Read the model definition and answer for the solid it produces. Units are mm, in the model's axes. A direction names the side the tool comes from. Round coordinates to 2 decimals unless told otherwise and drop trailing zeros. Order: outer loops, then holes, each group sorted by start corner. A loop starts at its lowest first (then second) coordinate and runs counter-clockwise, first axis right, second up. Notation, with made-up numbers: (68, 37.25) -> (89, 37.25) arc R11 cw to (89, 54.25) -> close; hole circle Ø7 at (63, -32.75). An arc over 180 degrees is marked (long way). Answer as a JSON object with one key per item and string values. Group by question number.
Item 1: Given P1, Ø11.5, axis at x = 18, z = -9, coming from the +Y side; P2, Ø6, axis at x = 160.5, z = -59.5, coming from the -Y side, each flat-ended and moving along its own axis, determine where each tip first touches the part or whether it passes through.
Item 2: For faces 1 (the flat face through (16.328, 2.421, -36.696)), 2 (the cylindrical face through (139.773, 10.988, -4.93)), 3 (the flat face through (178, 13, -9)), determine the directions among +Z, -Z, +X, -X, +Y, -Y from which every point of the face is accessible in a straight line to the end or side of a thin tool.
Item 3: The mould has two halves that part along X. Classify faces 4 (the flat face through (3, 15.2, -103.9)), 5 (the flat face through (16, 12.4, -34)), 6 (the flat face through (97, 0, -30)): pulls with the +X half, pulls with the -X half, needs draft (parallel to the pull), parting line crosses it, or undercut.
Item 4: Section C-C, the plane x = 68 is taken. Write down the section's boundary in (y, z).
Item 5: Section B-B, the plane y = 17.5 is taken. Count the separate pieces of the cut face and the enclosed holes in it, plus the area to 3 significant figures.
Item 6: Section D-D, the plane z = -73 is taken. Write down the section's boundary in (x, y) (3 decimals), plus the area to 3 significant figures.
Item 7: Section A-A, the plane x = 178 is taken. Write down the section's boundary in (y, z), plus the area to 3 significant figures.
Item 8: Consider probe 1 along X at (y, z) = (15, -53); probe 2 along X at (y, z) = (20, -98); probe 3 along Z at (x, y) = (138.5, 2.25). Determine where each line is inside the solid, lowest interval first. Write a range as from..to.
from build123d import *

# Parameters (mm, degrees)
SKETCH1_W            = 197
SKETCH1_H            = 107
BOSS_EXTRUDE1_DEPTH  = 30
SKETCH4_W            = 182
SKETCH4_H            = 45
CUT_EXTRUDE2_DEPTH   = 10
BOSS_EXTRUDE11_DEPTH = 10
CUT_EXTRUDE28_DEPTH  = 14.5
SKETCH9_R            = 8
CUT_EXTRUDE6_DEPTH   = 171
SKETCH10_R           = 9.5
CUT_EXTRUDE7_DEPTH   = 1.5
SKETCH11_R           = 4.95
CUT_EXTRUDE8_DEPTH   = 17.6
SKETCH41_R           = 2.9
CUT_EXTRUDE21_DEPTH  = 7
CUT_EXTRUDE22_DEPTH  = 10
CUT_EXTRUDE23_DEPTH  = 10
CUT_EXTRUDE29_DEPTH  = 14.5
CUT_EXTRUDE36_DEPTH  = 55.4
SKETCH90_R           = 6.35
CUT_EXTRUDE38_DEPTH  = 17
SKETCH91_W           = 141.2
SKETCH91_H           = 21.2
CUT_EXTRUDE39_DEPTH  = 2.3
CUT_EXTRUDE40_DEPTH  = 227.181343174


with BuildPart() as part:
    # Sketch1 → Boss-Extrude1 (new body)
    with BuildSketch(Plane(origin=(0, 0, 0), x_dir=(1, 0, 0), z_dir=(0, 1, 0))):
        with Locations((98.5, 53.5)):
            Rectangle(SKETCH1_W, SKETCH1_H)
    extrude(amount=BOSS_EXTRUDE1_DEPTH)

    # Sketch4 → Cut-Extrude2 (cut)
    with BuildSketch(Plane(origin=(0, 0, 0), x_dir=(1, 0, 0), z_dir=(0, 1, 0))):
        with Locations((98.5, 53.5)):
            Rectangle(SKETCH4_W, SKETCH4_H)
    extrude(amount=CUT_EXTRUDE2_DEPTH, mode=Mode.SUBTRACT)

    # Sketch53 → Boss-Extrude11 (add)
    with BuildSketch(Plane(origin=(0, 10, 0), x_dir=(-1, 0, 0), z_dir=(0, -1, 0))):
        Polygon((-7.5, 51), (-7.5, 31), (-38.5, 31), align=None)
        Polygon((-7.5, 56), (-7.5, 76), (-38.5, 76), align=None)
    extrude(amount=BOSS_EXTRUDE11_DEPTH)

    # Izq → Cut-Extrude28 (cut)
    with BuildSketch(Plane(origin=(0, 27.358390683, -11.62731604), x_dir=(1, 0, 0), z_dir=(0, 0.9203309184584746, -0.3911406403448515))):
        Polygon((7.5, 48.213835991), (38.5, 69.945149803), (7.5, 69.945149803), align=None)
    extrude(amount=-CUT_EXTRUDE28_DEPTH, mode=Mode.SUBTRACT)

    # Sketch9 → Cut-Extrude6 (cut)
    with BuildSketch(Plane(origin=(0, 30, 0), x_dir=(1, 0, 0), z_dir=(0, 1, 0))):
        with Locations(Location((15.45, 53.5, 0), (0, 0, 270))):
            Circle(SKETCH9_R)
    extrude(amount=-CUT_EXTRUDE6_DEPTH, mode=Mode.SUBTRACT)

    # Sketch10 → Cut-Extrude7 (cut)
    with BuildSketch(Plane(origin=(0, 30, 0), x_dir=(1, 0, 0), z_dir=(0, 1, 0))):
        with Locations(Location((15.45, 53.5, 0), (0, 0, 270))):
            Circle(SKETCH10_R)
    extrude(amount=-CUT_EXTRUDE7_DEPTH, mode=Mode.SUBTRACT)

    # Sketch11 → Cut-Extrude8 (cut)
    with BuildSketch(Plane(origin=(0, 30, 0), x_dir=(1, 0, 0), z_dir=(0, 1, 0))):
        with Locations(Location((15.45, 72.905102572, 0), (0, 0, 270))):
            Circle(SKETCH11_R)
        with Locations(Location((15.45, 34.094897428, 0), (0, 0, 270))):
            Circle(SKETCH11_R)
    extrude(amount=-CUT_EXTRUDE8_DEPTH, mode=Mode.SUBTRACT)

    # Sketch41 → Cut-Extrude21 (cut)
    with BuildSketch(Plane(origin=(0, 0, 0), x_dir=(1, 0, 0), z_dir=(0, 1, 0))):
        with Locations(Location((138.5, 9, 0), (0, 0, 90))):
            Circle(SKETCH41_R)
        with Locations(Location((138.5, 98, 0), (0, 0, 90))):
            Circle(SKETCH41_R)
    extrude(amount=CUT_EXTRUDE21_DEPTH, mode=Mode.SUBTRACT)

    # Sketch42 → Cut-Extrude22 (cut)
    with BuildSketch(Plane.XY):
        with BuildLine():
            Line((141.261527075, 12.77273886), (151, 12.77273886))
            ThreePointArc((151, 12.77273886), (152.77273886, 11), (151, 9.22726114))
            Line((151, 9.22726114), (141.261527075, 9.27273886))
            ThreePointArc((141.261527075, 9.27273886), (139.77273886, 11.02273886), (141.261527075, 12.77273886))
        make_face()
    extrude(amount=-CUT_EXTRUDE22_DEPTH, mode=Mode.SUBTRACT)

    # Sketch43 → Cut-Extrude23 (cut)
    with BuildSketch(Plane(origin=(0, 0, -107), x_dir=(-1, 0, 0), z_dir=(0, 0, -1))):
        with BuildLine():
            Line((-55.7, 12.8), (-46, 12.8))
            ThreePointArc((-46, 12.8), (-44.2, 11), (-46, 9.2))
            Line((-46, 9.2), (-55.7, 9.2))
            ThreePointArc((-55.7, 9.2), (-57.5, 11), (-55.7, 12.8))
        make_face()
    extrude(amount=-CUT_EXTRUDE23_DEPTH, mode=Mode.SUBTRACT)

    # Der → Cut-Extrude29 (cut)
    with BuildSketch(Plane(origin=(0, -11.159343568, -4.742721016), x_dir=(1, 0, 0), z_dir=(0, 0.9203309184584747, 0.3911406403448517))):
        Polygon((7.5, 50.261572284), (38.5, 28.530258472), (7.5, 28.530258472), align=None)
    extrude(amount=-CUT_EXTRUDE29_DEPTH, mode=Mode.SUBTRACT)

    # Sketch85 → Cut-Extrude36 (cut)
    with BuildSketch(Plane(origin=(0, 30, 0), x_dir=(1, 0, 0), z_dir=(0, 1, 0))):
        Polygon((0, 100.9), (6.1, 107), (0, 107), align=None)
        Polygon((0, 0), (6.1, 0), (0, 6.1), align=None)
        Polygon((197, 6.1), (190.9, 0), (197, 0), align=None)
        Polygon((197, 107), (190.9, 107), (197, 100.9), align=None)
    extrude(amount=-CUT_EXTRUDE36_DEPTH, mode=Mode.SUBTRACT)

    # Sketch90 → Cut-Extrude38 (cut)
    with BuildSketch(Plane(origin=(0, 30, 0), x_dir=(1, 0, 0), z_dir=(0, 1, 0))):
        with Locations(Location((18, 9, 0), (0, 0, 270))):
            Circle(SKETCH90_R)
        with Locations(Location((98, 9, 0), (0, 0, 270))):
            Circle(SKETCH90_R)
        with Locations(Location((178, 9, 0), (0, 0, 270))):
            Circle(SKETCH90_R)
        with Locations(Location((98, 98, 0), (0, 0, 270))):
            Circle(SKETCH90_R)
        with Locations(Location((178, 98, 0), (0, 0, 270))):
            Circle(SKETCH90_R)
        with Locations(Location((18, 98, 0), (0, 0, 270))):
            Circle(SKETCH90_R)
    extrude(amount=-CUT_EXTRUDE38_DEPTH, mode=Mode.SUBTRACT)

    # Sketch91 → Cut-Extrude39 (cut)
    with BuildSketch(Plane(origin=(0, 30, 0), x_dir=(1, 0, 0), z_dir=(0, 1, 0))):
        with BuildLine():
            Line((42.6, 66.5), (182.6, 66.5))
            ThreePointArc((182.6, 66.5), (184.721320344, 65.621320344), (185.6, 63.5))
            Line((185.6, 63.5), (185.6, 43.5))
            ThreePointArc((185.6, 43.5), (184.721320344, 41.378679656), (182.6, 40.5))
            Line((182.6, 40.5), (42.6, 40.5))
            ThreePointArc((42.6, 40.5), (40.478679656, 41.378679656), (39.6, 43.5))
            Line((39.6, 43.5), (39.6, 63.5))
            ThreePointArc((39.6, 63.5), (40.478679656, 65.621320344), (42.6, 66.5))
        make_face()
        with Locations((112.6, 53.5)):
            Rectangle(SKETCH91_W, SKETCH91_H, mode=Mode.SUBTRACT)
    extrude(amount=-CUT_EXTRUDE39_DEPTH, mode=Mode.SUBTRACT)

    # Sketch93 → Cut-Extrude40 (cut, through all)
    with BuildSketch(Plane(origin=(0, 30, 0), x_dir=(1, 0, 0), z_dir=(0, 1, 0))):
        with BuildLine():
            Line((45.1, 43.5), (180.1, 43.5))
            ThreePointArc((180.1, 43.5), (181.867766953, 44.232233047), (182.6, 46))
            Line((182.6, 46), (182.6, 61))
            ThreePointArc((182.6, 61), (181.867766953, 62.767766953), (180.1, 63.5))
            Line((180.1, 63.5), (45.1, 63.5))
            ThreePointArc((45.1, 63.5), (43.332233047, 62.767766953), (42.6, 61))
            Line((42.6, 61), (42.6, 46))
            ThreePointArc((42.6, 46), (43.332233047, 44.232233047), (45.1, 43.5))
        make_face()
    extrude(amount=-CUT_EXTRUDE40_DEPTH, mode=Mode.SUBTRACT)


solid = part.part
Values found:
{
 "1": {"P1": "y = 13", "P2": "through"},
 "2": {"face 1": "-Y", "face 2": "+Z", "face 3": "+Y"},
 "3": {"face 4": "pulls with the -X half", "face 5": "undercut", "face 6": "needs draft"},
 "4": {"outline": "(0, -107) -> (30, -107) -> (30, -66.5) -> (27.7, -66.5) -> (27.7, -64.1) -> (30, -64.1) -> (30, -63.5) -> (10, -63.5) -> (10, -76) -> (0, -76) -> close; (0, -31) -> (10, -31) -> (10, -43.5) -> (30, -43.5) -> (30, -42.9) -> (27.7, -42.9) -> (27.7, -40.5) -> (30, -40.5) -> (30, 0) -> (0, 0) -> close"},
 "5": {"separate pieces": "1", "enclosed holes": "10", "area": "17,100 mm2"},
 "6": {"outline": "(0, 0) -> (7.5, 0) -> (7.5, 1.275) -> (33.85, 1.275) -> (33.85, 10) -> (189.5, 10) -> (189.5, 0) -> (197, 0) -> (197, 30) -> (20.399, 30) -> (20.399, 12.4) -> (10.501, 12.4) -> (10.501, 30) -> (0, 30) -> close", "area": "4,150 mm2"},
 "7": {"outline": "(0, -107) -> (30, -107) -> (30, -104.35) -> (13, -104.35) -> (13, -91.65) -> (30, -91.65) -> (30, -66.5) -> (27.7, -66.5) -> (27.7, -64.1) -> (30, -64.1) -> (30, -63.5) -> (10, -63.5) -> (10, -76) -> (0, -76) -> close; (0, -31) -> (10, -31) -> (10, -43.5) -> (30, -43.5) -> (30, -42.9) -> (27.7, -42.9) -> (27.7, -40.5) -> (30, -40.5) -> (30, -15.35) -> (13, -15.35) -> (13, -2.65) -> (30, -2.65) -> (30, 0) -> (0, 0) -> close", "area": "1,920 mm2"},
 "8": {"probe 1": "0..7.47, 23.43..42.6, 182.6..197", "probe 2": "0..11.65, 24.35..91.65, 104.35..171.65, 184.35..197", "probe 3": "-107..-100.9, -95.1..-76, -31..-11.9, -6.1..0"}
}
